For this review, use the dimensioned drawing (mm, ordinates from the lowest corner) and the shaded views. A direction names the side the tool comes from. Round coordinates to 2 decimals unless told otherwise and drop trailing zeros. Loops run counter-clockwise (first coordinate to the right, second up) from the corner with the lowest first, then second, coordinate; pieces in that order, holes last. Notation, with made-up numbers: (18, -28) -> (62, -28) arc R27 ccw to (62, 2) -> close; hole circle Ø3 at (27.25, 49). An arc over 180 degrees is marked (long way). Answer as CSV lines item,"result". Start each with the question number.
(1) Take a section at D-D, the plane y = 52. Write out the cut boundary in (x, z) (1 decimal), and give its area (3 significant figures).
(2) Take a section at A-A, the plane z = 22. Write out the cut boundary in (x, y) (1 decimal).
(3) To check wall thickness, follow line 1 (Z direction, x = 22.5, y = 38); line 2 (X direction, y = 49.5, z = 15) (1 decimal); line 3 (X direction, y = 55, z = 17) (1 decimal). State the ranges of each line that lie inside material, in increasing order. Write a range as from..to.
(4) Take a section at C-C, the plane x = 49. Write out the cut boundary in (y, z) (1 decimal).
(5) Take a section at B-B, the plane y = 69.5. Write out the cut boundary in (x, z) (1 decimal), and give its area (3 significant figures).
(6) Draft analysis for pull direction X (two halves, no side actions). For the marked faces 3, 4, 5 and 6, state which applies: +X half, -X half, draft (parallel to the pull), parting line (faces both ways), or undercut.
(7) Machinability: for the marked faces 1 and 2, which of the approach directions +Z, -Z, +X, -X, +Y, -Y give a long, thin tool a straight path to every point of the face, cutting with its end or side? Answer none if there is none.
(8) For P1, Ø2, axis at x = 51.5, y = 38, coming from the +Z side; P2, Ø8, axis at x = 27.5, y = 59, coming from the -Z side, all flat-tipped, find the tip position at first contact; note any pin that passes through.
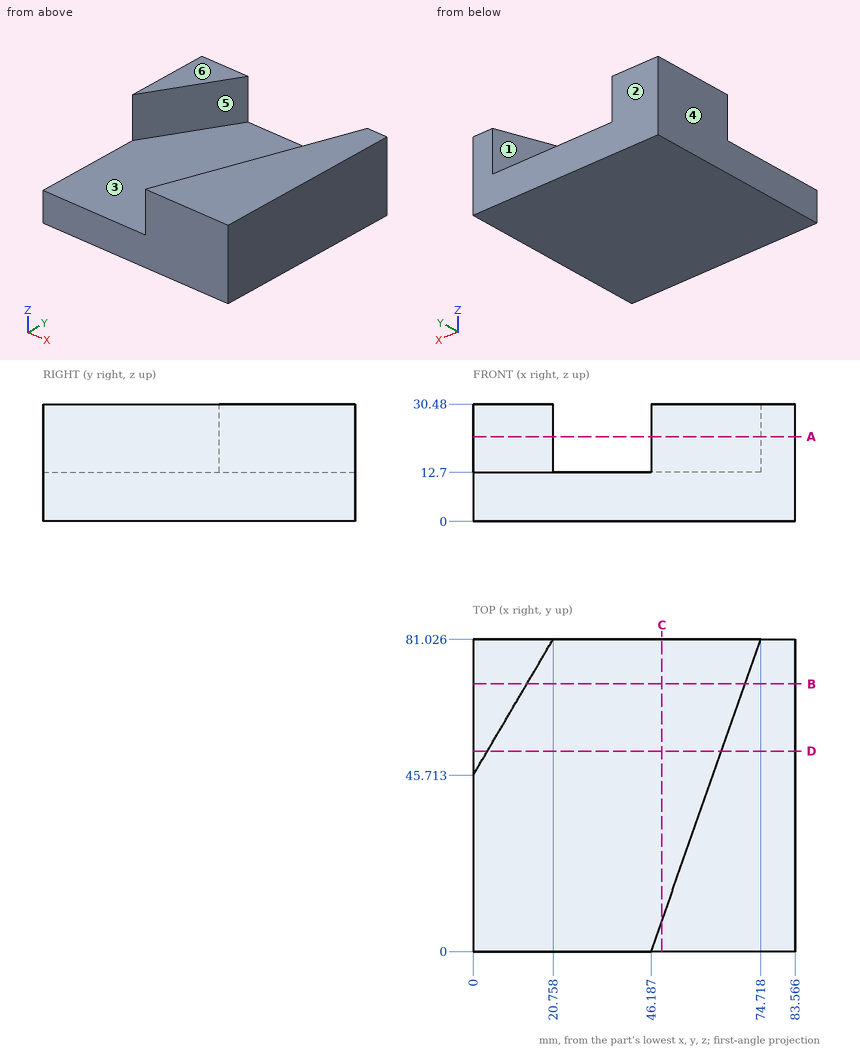
The answers:
1,outline,"(0, 0) -> (83.6, 0) -> (83.6, 30.5) -> (64.5, 30.5) -> (64.5, 12.7) -> (3.7, 12.7) -> (3.7, 30.5) -> (0, 30.5) -> close"
1,area,"1,470 mm²"
2,outline,"(0, 45.7) -> (20.8, 81) -> (0, 81) -> close; (46.2, 0) -> (83.6, 0) -> (83.6, 81) -> (74.7, 81) -> close"
3,line 1,"0..12.7"
3,line 2,"0..2.2, 63.6..83.6"
3,line 3,"0..5.5, 65.6..83.6"
4,outline,"(0, 0) -> (81, 0) -> (81, 12.7) -> (8, 12.7) -> (8, 30.5) -> (0, 30.5) -> close"
5,outline,"(0, 0) -> (83.6, 0) -> (83.6, 30.5) -> (70.7, 30.5) -> (70.7, 12.7) -> (14, 12.7) -> (14, 30.5) -> (0, 30.5) -> close"
5,area,"1,540 mm²"
6,face 3,"undercut"
6,face 4,"-X half"
6,face 5,"undercut"
6,face 6,"draft"
7,face 1,"+Z, +Y"
7,face 2,"+Z, -Z, +X, -X, +Y"
8,P1,"z = 12.7"
8,P2,"z = 0"
